from build123d import *

# Parameters (mm, degrees)
F0_W     = 1422.4
F0_H     = 1422.4
F1_DEPTH = 28.575
F2_R     = 53.878299
F2_R_2   = 61.704348
F2_R_3   = 59.410664
F2_R_4   = 61.388417
F3_DEPTH = 127
F4_R     = 29.44728
F4_R_2   = 25.298259
F4_R_3   = 30.573071
F4_R_4   = 27.370078
F5_DEPTH = 428.45566
F6_R     = 124.806137
F7_DEPTH = 511.49744


with BuildPart() as f1:
    # F0 (on Top) → F1 (new body)
    with BuildSketch(Plane.XY):
        with Locations((-13.414681, 358.960475)):
            Rectangle(F0_W, F0_H)
    extrude(amount=F1_DEPTH)

    # F2 (on face) → F3 (join)
    with BuildSketch(Plane(origin=(0, 0, 0), x_dir=(1, 0, 0), z_dir=(0, 0, -1))):
        with Locations((591.243267, 266.280264)):
            Circle(F2_R)
        with Locations((591.243267, -976.189792)):
            Circle(F2_R_2)
        with Locations((-632.192075, -976.189792)):
            Circle(F2_R_3)
        with Locations((-632.192075, 266.280264)):
            Circle(F2_R_4)
    extrude(amount=F3_DEPTH)

    # F4 (on face) → F5 (cut)
    with BuildSketch(Plane.XY.offset(28.575)):
        with Locations((296.321899, 708.59462)):
            Circle(F4_R)
        with Locations((-455.202579, 708.59462)):
            Circle(F4_R_2)
        with Locations((-455.202579, -59.054408)):
            Circle(F4_R_3)
        with Locations((296.321899, -59.054408)):
            Circle(F4_R_4)
    extrude(amount=-F5_DEPTH, mode=Mode.SUBTRACT)

    # F6 (on face) → F7 (cut)
    with BuildSketch(Plane.XY.offset(28.575)):
        with Locations((-83.842769, -101.621295)):
            Circle(F6_R)
    extrude(amount=-F7_DEPTH, mode=Mode.SUBTRACT)


solid = f1.part
Read the model definition and answer for the solid it produces. Units are mm, in the model's axes. A direction names the side the tool comes from. Coordinates: 2 decimals unless noted, no trailing zeros. Write each loop counter-clockwise with the first axis right and the second up, starting at its lowest first coordinate (ties: lowest second). Pieces come first, ordered by that corner, then holes. Notation, with made-up numbers: M 11,54 L 35,54 A22 ccw 35,84 Z; hole C 42,8 d1. An arc over 180 degrees is marked long. Use a Markdown table: item, result.
Q1. The part is cut by section B-B, the plane y = -157. Write down the section's boundary in (x, z) (3 decimals), then the cut area to 3 significant figures.
Answer block:
| item | result |
|---|---|
| outline | M -724.615,0 L -195.69,0 L -195.69,28.575 L -724.615,28.575 Z; M 28.004,0 L 697.785,0 L 697.785,28.575 L 28.004,28.575 Z |
| area | 34,300 mm2 |
Q2. This flat-tipped pin is pushed along its axis until it touches: pin 1 Ø1.5 at (x, y) = (-284.5, 712) entering from -Z. Where does it stop, or does it pass through?
Answer block:
| item | result |
|---|---|
| pin 1 | stops at z = 0 |
Q3. Determine the mould class of faces 1 (the face through (-633, -267, -127)), 2 (the face through (-426.96, -70.76, 14.49)) for opening direction X: released by +X, released by -X, zero draft, split by the parting line, or undercut.
Answer block:
| item | result |
|---|---|
| face 1 | zero draft |
| face 2 | undercut |
Q4. The part is cut by section D-D, the plane x = 610. Write down the section's boundary in (y, z) (3 decimals), then the cut area to 3 significant figures.
Answer block:
| item | result |
|---|---|
| outline | M -352.24,0 L -316.788,0 L -316.788,-127 L -215.772,-127 L -215.772,0 L 917.405,0 L 917.405,-127 L 1034.974,-127 L 1034.974,0 L 1070.16,0 L 1070.16,28.575 L -352.24,28.575 Z |
| area | 68,400 mm2 |
Q5. Straight lines are drawn through the part: L1, parallel to Y at x = 590, z = -95; L2, parallel to Y at x = -629.5, z = -72.5; L3, parallel to Z at x = -214, y = 849.5 (3 decimals). For each, find the intervals that lie inside material, in ascending order. Write a range as [from, to].
Answer block:
| item | result |
|---|---|
| L1 | y = [-320.14, -212.42], [914.5, 1037.88] |
| L2 | y = [-327.61, -204.95], [916.84, 1035.54] |
| L3 | z = [0, 28.575] |
Q6. The part is cut by section A-A, the plane x = -185.5. Write down the section's boundary in (y, z) (3 decimals).
Answer block:
| item | result |
|---|---|
| outline | M -352.24,0 L -174.026,0 L -174.026,28.575 L -352.24,28.575 Z; M -29.217,0 L 1070.16,0 L 1070.16,28.575 L -29.217,28.575 Z |
Q7. The part is cut by section C-C, the plane z = -24. Write down the section's boundary in (x, y), then the cut area to 3 significant figures.
Answer block:
| item | result |
|---|---|
| outline | C -632.19,-266.28 d122.78; C -632.19,976.19 d118.82; C 591.24,976.19 d123.41; C 591.24,-266.28 d107.76 |
| area | 44,000 mm2 |
Q8. Which of the six approach directions +Z, -Z, +X, -X, +Y, -Y give full straight-line access (tool end or side, diameter ignored) to faces 3 (the face through (590, 975, -127)), 4 (the face through (-693.52, -268.98, -62.61))?
Answer block:
| item | result |
|---|---|
| face 3 | -Z, +X, -X, +Y, -Y |
| face 4 | -Z |
